from build123d import *

# Parameters (mm, degrees)
SKETCH_1_R      = 0.512380356
EXTRUDE_1_DEPTH = 0.4


with BuildPart() as part:
    # Эскиз1 → Бобышка-Вытянуть1 (new, symmetric)
    with BuildSketch(Plane(origin=(0, 0, 0), x_dir=(1, 0, 0), z_dir=(0, 1, 0))):
        Polygon((0, -2.467893219), (0, 2.467893219), (0.707106781, 3.175), (7.7, 3.175), (7.7, 3.95), (10.3, 3.95), (10.3, 3.225), (14, 3.225), (14, 1.875), (9.5, 1.875), (9.5, -1.875), (14, -1.875), (14, -3.225), (10.3, -3.225), (10.3, -3.95), (7.7, -3.95), (7.7, -3.175), (0.707106781, -3.175), align=None)
        with Locations(Location((1.761903111, 0, 0), (0, 0, 270))):
            Circle(SKETCH_1_R, mode=Mode.SUBTRACT)
    extrude(amount=EXTRUDE_1_DEPTH, both=True)


solid = part.part
Geometry check sheet. Reference: the model listing, model coordinates, mm. Coordinates: 2 decimals unless noted, no trailing zeros. Order: outer loops, then holes, each group sorted by start corner. A loop starts at its lowest first (then second) coordinate and runs counter-clockwise, first axis right, second up. Notation, with made-up numbers: (-16.5, 18) -> (20.5, 18) arc R21 cw to (20.5, 50) -> close; hole circle Ø7 at (85.25, 27). An arc over 180 degrees is marked (long way). Use a Markdown table: item, result. Add a question column.
1. Cross-section at A-A (x = 13). Enter the section's corners in (y, z) (3 decimals).
2. Cross-section at B-B (z = 0). Enter the section's corners in (x, y).
3. Mould release check, pull along Z, two halves, no side actions. Record for faces 1 (the face through (2.19, -0.01, 0.28)), 2 (the face through (6, -0.4, 0)): pulls with the +Z half, pulls with the -Z half, needs draft (parallel to the pull), parting line crosses it, or undercut.
4. Material ranges on L1, parallel to Z at x = 10.5, y = -0.25 (3 decimals); L2, parallel to X at y = 0.25, z = 0; L3, parallel to X at y = -0.15, z = 1.25, recorded low to high.
5. Cross-section at C-C (y = 0.1). Enter the section's corners in (x, z) (3 decimals), and give its area (3 significant figures).
6. Cross-section at D-D (x = 7.5). Enter the section's corners in (y, z) (3 decimals).
Filled sheet:
| question | item | result |
|---|---|---|
| 1 | outline | (-0.4, -3.225) -> (0.4, -3.225) -> (0.4, -1.875) -> (-0.4, -1.875) -> close; (-0.4, 1.875) -> (0.4, 1.875) -> (0.4, 3.225) -> (-0.4, 3.225) -> close |
| 2 | outline | (0, -0.4) -> (1.25, -0.4) -> (1.25, 0.4) -> (0, 0.4) -> close; (2.27, -0.4) -> (9.5, -0.4) -> (9.5, 0.4) -> (2.27, 0.4) -> close |
| 3 | face 1 | undercut |
| 3 | face 2 | needs draft |
| 4 | L1 | -3.225 to -1.875, 1.875 to 3.225 |
| 4 | L2 | 0 to 1.25, 2.27 to 9.5 |
| 4 | L3 | 0 to 9.5 |
| 5 | outline | (0, -2.468) -> (0.707, -3.175) -> (7.7, -3.175) -> (7.7, -3.95) -> (10.3, -3.95) -> (10.3, -3.225) -> (14, -3.225) -> (14, -1.875) -> (9.5, -1.875) -> (9.5, 1.875) -> (14, 1.875) -> (14, 3.225) -> (10.3, 3.225) -> (10.3, 3.95) -> (7.7, 3.95) -> (7.7, 3.175) -> (0.707, 3.175) -> (0, 2.468) -> close; hole circle Ø1.025 at (1.762, 0) |
| 5 | area | 75.1 mm2 |
| 6 | outline | (-0.4, -3.175) -> (0.4, -3.175) -> (0.4, 3.175) -> (-0.4, 3.175) -> close |
